from build123d import *

# Parameters (mm, degrees)
SKETCH1_W           = 104.902
SKETCH1_H           = 114.3
BOSS_EXTRUDE1_DEPTH = 6.35
CUT_EXTRUDE2_REACH  = 79.83
SKETCH3_R           = 3.429
CUT_EXTRUDE3_REACH  = 79.83
SKETCH4_R           = 7.9375


with BuildPart() as part:
    # Sketch1 → Boss-Extrude1 (new body)
    with BuildSketch(Plane(origin=(0, 0, 0), x_dir=(1, 0, 0), z_dir=(0, 1, 0))):
        Rectangle(SKETCH1_W, SKETCH1_H)
    extrude(amount=BOSS_EXTRUDE1_DEPTH)

    # Sketch3 → Cut-Extrude2 (cut, up to next)
    with BuildSketch(Plane.XZ, mode=Mode.PRIVATE) as cut_extrude2_sk1:
        with Locations(Location((-33.528, 37.846, 0), (0, 0, 270))):
            Circle(SKETCH3_R)
    cut_extrude2_tool1 = extrude(cut_extrude2_sk1.sketch, amount=-CUT_EXTRUDE2_REACH, mode=Mode.PRIVATE) & part.part
    # Sketch3 → Cut-Extrude2 (cut, up to next)
    with BuildSketch(Plane.XZ, mode=Mode.PRIVATE) as cut_extrude2_sk2:
        with Locations(Location((-33.528, -37.846, 0), (0, 0, 90))):
            Circle(SKETCH3_R)
    cut_extrude2_tool2 = extrude(cut_extrude2_sk2.sketch, amount=-CUT_EXTRUDE2_REACH, mode=Mode.PRIVATE) & part.part
    # Sketch3 → Cut-Extrude2 (cut, up to next)
    with BuildSketch(Plane.XZ, mode=Mode.PRIVATE) as cut_extrude2_sk3:
        with Locations(Location((36.068, 37.846, 0), (0, 0, 90))):
            Circle(SKETCH3_R)
    cut_extrude2_tool3 = extrude(cut_extrude2_sk3.sketch, amount=-CUT_EXTRUDE2_REACH, mode=Mode.PRIVATE) & part.part
    # Sketch3 → Cut-Extrude2 (cut, up to next)
    with BuildSketch(Plane.XZ, mode=Mode.PRIVATE) as cut_extrude2_sk4:
        with Locations(Location((36.068, -37.846, 0), (0, 0, 270))):
            Circle(SKETCH3_R)
    cut_extrude2_tool4 = extrude(cut_extrude2_sk4.sketch, amount=-CUT_EXTRUDE2_REACH, mode=Mode.PRIVATE) & part.part
    add(cut_extrude2_tool1.solids().sort_by_distance((-33.528, 0, 37.846))[0], mode=Mode.SUBTRACT)
    add(cut_extrude2_tool2.solids().sort_by_distance((-33.528, 0, -37.846))[0], mode=Mode.SUBTRACT)
    add(cut_extrude2_tool3.solids().sort_by_distance((36.068, 0, 37.846))[0], mode=Mode.SUBTRACT)
    add(cut_extrude2_tool4.solids().sort_by_distance((36.068, 0, -37.846))[0], mode=Mode.SUBTRACT)

    # Sketch4 → Cut-Extrude3 (cut, up to next)
    with BuildSketch(Plane.XZ, mode=Mode.PRIVATE) as cut_extrude3_sk1:
        with Locations(Location((0, 0, 0), (0, 0, 270))):
            Circle(SKETCH4_R)
    cut_extrude3_tool1 = extrude(cut_extrude3_sk1.sketch, amount=-CUT_EXTRUDE3_REACH, mode=Mode.PRIVATE) & part.part
    add(cut_extrude3_tool1.solids().sort_by_distance((0, 0, 0))[0], mode=Mode.SUBTRACT)


solid = part.part
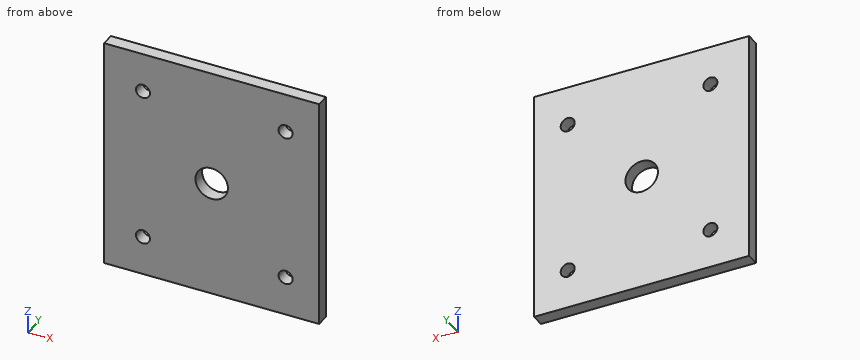
For this review, take the finished solid that the model builds, in its own axes (mm). Round coordinates to 2 decimals unless told otherwise and drop trailing zeros. Loops run counter-clockwise (first coordinate to the right, second up) from the corner with the lowest first, then second, coordinate; pieces in that order, holes last. Notation, with made-up numbers: (36, 45.5) - (88, 45.5) arc R26 cw to (88, 81.5) - close; hole circle Ø11 at (70, 49.25). An arc over 180 degrees is marked (long way). Answer as CSV lines item,"result".
(1) Consider section A-A on x = 0. Give the boundary of the cut face in (y, z).
Checked values:
outline,"(0, -57.15) - (6.35, -57.15) - (6.35, -7.94) - (0, -7.94) - close; (0, 7.94) - (6.35, 7.94) - (6.35, 57.15) - (0, 57.15) - close"
(2) Consider section D-D on x = -32. Give the boundary of the cut face in (y, z), then the cut area to 3 significant figures.
Checked values:
outline,"(0, -57.15) - (6.35, -57.15) - (6.35, -40.92) - (0, -40.92) - close; (0, -34.78) - (6.35, -34.78) - (6.35, 34.78) - (0, 34.78) - close; (0, 40.92) - (6.35, 40.92) - (6.35, 57.15) - (0, 57.15) - close"
area,"648 mm2"
(3) Consider section B-B on z = 0. Give the boundary of the cut face in (x, y), then the cut area to 3 significant figures.
Checked values:
outline,"(-52.45, 0) - (-7.94, 0) - (-7.94, 6.35) - (-52.45, 6.35) - close; (7.94, 0) - (52.45, 0) - (52.45, 6.35) - (7.94, 6.35) - close"
area,"565 mm2"
(4) Insertion check: P1, Ø11, axis at x = 36.068, z = 37.846, coming from the -Y side. The pin has a flat end and moves straight along its axis. Give the tip position at first contact, or say it passes through.
Checked values:
P1,"stops at y = 0"
(5) Wall thickness on line 1 (X direction, y = 2.25, z = -37.5); line 2 (Z direction, x = 39, y = 4); line 3 (X direction, y = 5.5, z = -0.5): over which ranges is each line inside the solid? List them lowest first.
Checked values:
line 1,"x = -52.45 to -36.94, -30.12 to 32.66, 39.48 to 52.45"
line 2,"z = -57.15 to -39.62, -36.07 to 36.07, 39.62 to 57.15"
line 3,"x = -52.45 to -7.92, 7.92 to 52.45"
(6) Consider section C-C on y = 4.5. Give the number of separate pieces and of enclosed holes in the cut face, then the cut area to 3 significant figures.
Checked values:
separate pieces,"1"
enclosed holes,"5"
area,"11,600 mm2"
